Geometry: final body of the model. Coordinates: model frame, mm. A direction names the side the tool comes from. Give positions to 0.01 mm unless a question says otherwise; leave off trailing zeros. Write each loop counter-clockwise with the first axis right and the second up, starting at its lowest first coordinate (ties: lowest second). Pieces come first, ordered by that corner, then holes. Notation, with made-up numbers: (-35, 34) -> (8, 34) arc R16 cw to (8, 61) -> close; hole circle Ø2 at (86, -23.5). An arc over 180 degrees is marked (long way). Answer as a JSON object with one key per item and string values. Group by question number.
(1) Set-up query: faces 1 (the face through (42, 2, 0)), 2 (the face through (2.27, -3.04, -3.32)), 3 (the face through (1.183, -1.293, -0.76)). Return all of +Z, -Z, +X, -X, +Y, -Y with unobstructed straight access to the full face (end or side cutting, diameter ignored); none if empty.
(2) Section query C-C on x = 9. Output: boundary loops of the cut face in (y, z).
(3) Draft query along Z for faces 4 (the face through (21.2, -0.1, -2.5)), 5 (the face through (1.183, 1.305, -0.74)), 6 (the face through (3.5, 2, 2)). Return one class per face: +Z half, -Z half, draft (parallel to the pull), parting line (faces both ways), or undercut.
(4) Material intervals for probe 1 along X at (y, z) = (0.75, 2.75); probe 2 along Y at (x, z) = (5.5, 1.5); probe 3 along Y at (x, z) = (5, 2), sorted ascending.
(5) Section query A-A on y = 0. Output: boundary loops of the cut face in (x, z).
(6) Contact query for flat-ended pins moving along their axis: pin 1 Ø3 at (x, z) = (14.5, 2.5) entering from -Y; pin 2 Ø3 at (x, z) = (34, 0) entering from +Y; pin 3 Ø5 at (x, z) = (36, 3) entering from +Y. Output: stop coordinate, or through.
(7) Section query B-B on x = 40.5. Output: boundary loops of the cut face in (y, z), plus the area to 3 significant figures.
from build123d import *

# Parameters (mm, degrees)
CUT_EXTRUDE_1_DEPTH = 2.4
FILLET_1_R          = 1
CHAMFER_1_SIZE      = 0.5


with BuildPart() as part:
    # 草图1 → 旋转1 (revolve)
    with BuildSketch(Plane.XY, mode=Mode.PRIVATE) as revolve_1_sk:
        Polygon((0, 0), (0, 4.5), (3.5, 4.5), (3.5, 2.5), (38.5, 2.5), (38.5, 2), (46.5, 2), (46.5, 0), align=None)
    revolve(revolve_1_sk.sketch.rotate(Axis((0, 0, 0), (1, 0, 0)), 90), axis=Axis((0, 0, 0), (1, 0, 0)))

    # 草图2 → 切除-拉伸1 (cut)
    with BuildSketch(Plane.ZY):
        Polygon((0, 1.732050808), (-1.5, 0.866025404), (-1.5, -0.866025404), (0, -1.732050808), (1.5, -0.866025404), (1.5, 0.866025404), align=None)
    extrude(amount=-CUT_EXTRUDE_1_DEPTH, mode=Mode.SUBTRACT)

    # 圆角1
    fillet_1_edges = [part.edges().sort_by_distance(p)[0] for p in [
        (0, 0, -4.5),
    ]]
    fillet(fillet_1_edges, radius=FILLET_1_R)

    # 倒角1
    chamfer_1_edges = [part.edges().sort_by_distance(p)[0] for p in [
        (46.5, 0, -2),
    ]]
    chamfer(chamfer_1_edges, length=CHAMFER_1_SIZE)


solid = part.part
Answer list:
{
 "1": {"face 1": "+X", "face 2": "+X, -X", "face 3": "-X"},
 "2": {"outline": "circle Ø5 at (0, 0)"},
 "3": {"face 4": "parting line", "face 5": "undercut", "face 6": "draft"},
 "4": {"probe 1": "0 to 3.5", "probe 2": "-2 to 2", "probe 3": "-1.5 to 1.5"},
 "5": {"outline": "(0, -3.5) arc R1 ccw to (1, -4.5) -> (3.5, -4.5) -> (3.5, -2.5) -> (38.5, -2.5) -> (38.5, -2) -> (46, -2) -> (46.5, -1.5) -> (46.5, 1.5) -> (46, 2) -> (38.5, 2) -> (38.5, 2.5) -> (3.5, 2.5) -> (3.5, 4.5) -> (1, 4.5) arc R1 ccw to (0, 3.5) -> (0, 1.5) -> (2.4, 1.5) -> (2.4, -1.5) -> (0, -1.5) -> close"},
 "6": {"pin 1": "y = -2.29", "pin 2": "y = 2.5", "pin 3": "y = 2.45"},
 "7": {"outline": "circle Ø4 at (0, 0)", "area": "12.6 mm2"}
}
